```python
from build123d import *

# Parameters (mm, degrees)
BOSS_EXTRUDE1_DEPTH = 60
FILLET1_R           = 20
FILLET2_R           = 50
SKETCH2_W           = 946.025641026
SKETCH2_H           = 25
CUT_EXTRUDE1_DEPTH  = 1147.843494118
FILLET3_R           = 15
BOSS_EXTRUDE2_DEPTH = 60
CHAMFER1_START      = 58.356662002
CHAMFER1_OUTLINE_W  = 43
CHAMFER1_OUTLINE_H  = 66
CHAMFER1_DEPTH      = 20.643337998
CHAMFER2_START      = 58.356662002
CHAMFER2_OUTLINE_W  = 43
CHAMFER2_OUTLINE_H  = 66
CHAMFER2_DEPTH      = 20.643337998
FILLET4_R           = 1


with BuildPart() as part:
    # Sketch1 → Boss-Extrude1 (new, symmetric)
    with BuildSketch(Plane.XY):
        Polygon((0, 0), (0, -525), (-985, -525), (-985, -536), (-765, -575), (40, -575), (40, 0), align=None)
    extrude(amount=BOSS_EXTRUDE1_DEPTH, both=True)

    # Fillet1
    fillet1_edges = [part.edges().sort_by_distance(p)[0] for p in [
        (0, -525, 0),
    ]]
    fillet(fillet1_edges, radius=FILLET1_R)

    # Fillet2
    fillet2_edges = [part.edges().sort_by_distance(p)[0] for p in [
        (40, -575, 0),
    ]]
    fillet(fillet2_edges, radius=FILLET2_R)

    # Sketch2 → Cut-Extrude1 (cut, through all)
    with BuildSketch(Plane.XY.offset(60)):
        with Locations((-433.012820513, -562.5)):
            Rectangle(SKETCH2_W, SKETCH2_H)
    extrude(amount=-CUT_EXTRUDE1_DEPTH, mode=Mode.SUBTRACT)

    # Fillet3
    fillet3_edges = [part.edges().sort_by_distance(p)[0] for p in [
        (-985, -530.5, 60),
        (-985, -530.5, -60),
    ]]
    fillet(fillet3_edges, radius=FILLET3_R)

    # Sketch4 → Boss-Extrude2 (add, symmetric)
    with BuildSketch(Plane.XY):
        Polygon((40, -23), (71, -23), (71, -83), (62, -83), (56.90441672, -69), (40, -69), align=None)
        Polygon((40, -484), (51.812506017, -484), (58, -467), (70, -467), (70, -477), (60.172803675, -504), (40, -504), align=None)
    extrude(amount=BOSS_EXTRUDE2_DEPTH, both=True)

    # Chamfer1: read off the stored shape, not the designer's step
    # Chamfer1 outline → Chamfer1 (cut)
    with BuildSketch(Plane(origin=(0, 0, 0), x_dir=(0.7514973063417119, -0.31591606508632464, -0.5791794526582624), z_dir=(0.659736158294474, 0.35985608634244, 0.659736158294474)).offset(CHAMFER1_START)):
        with Locations((23.5, -66)):
            Rectangle(CHAMFER1_OUTLINE_W, CHAMFER1_OUTLINE_H)
    extrude(amount=CHAMFER1_DEPTH, mode=Mode.SUBTRACT)

    # Chamfer2: read off the stored shape, not the designer's step
    # Chamfer2 outline → Chamfer2 (cut)
    with BuildSketch(Plane(origin=(0, 0, 0), x_dir=(0.7514973063417119, -0.31591606508632464, 0.5791794526582624), z_dir=(0.659736158294474, 0.35985608634244, -0.659736158294474)).offset(CHAMFER2_START)):
        with Locations((23.5, 66)):
            Rectangle(CHAMFER2_OUTLINE_W, CHAMFER2_OUTLINE_H)
    extrude(amount=CHAMFER2_DEPTH, mode=Mode.SUBTRACT)

    # Fillet4
    fillet4_edges = [part.edges().sort_by_distance(p)[0] for p in [
        (56, -50.5, 60),
        (71, -23, 0),
        (71, -50.5, 45),
        (56, -23, 45),
        (56, -23, -45),
        (71, -50.5, -45),
        (56, -50.5, -60),
        (71, -83, 0),
        (40, -504, 0),
        (60.172803675, -504, 0),
        (70, -477, 0),
        (70, -467, 0),
    ]]
    fillet(fillet4_edges, radius=FILLET4_R)


solid = part.part
```
Build history of the part. All positions in model axes, mm. A direction names the side the tool comes from. Coordinates: 2 decimals unless noted, no trailing zeros. Order: outer loops, then holes, each group sorted by start corner. A loop starts at its lowest first (then second) coordinate and runs counter-clockwise, first axis right, second up.
Item 1: Tool access for faces 1 (the flat face through (-496, -525, 1)), 2 (the flat face through (40, -515, 1)), 3 (the flat face through (51, -23, -1)): list every direction of +Z, -Z, +X, -X, +Y, -Y with a clear straight run to the whole face (end or side of a thin tool).
Filled in:
face 1: +Z, -Z, -X, +Y
face 2: +Z, -Z, +X, -Y
face 3: +Z, -Z, +X, +Y
Item 2: Saw through at B-B on y = -345. List the corners of the cut face in (x, z), then the cut area to 3 significant figures.
Filled in:
outline: (0, -60) - (40, -60) - (40, 60) - (0, 60) - close
area: 4,800 mm2
Item 3: Drill centre lines: L1, parallel to X at y = -241, z = 27; L2, parallel to Y at x = -677.5, z = 0.5; L3, parallel to X at y = -57, z = -10. Where is each one in solid material? Low to high.
Filled in:
L1: x = 0 to 40
L2: y = -550 to -525
L3: x = 0 to 71
Item 4: Saw through at A-A on z = -14.5. List the corners of the cut face in (x, y), then the cut area to 3 significant figures.
Filled in:
outline: (-985, -536) - (-906.03, -550) - (33.3, -550) arc R50 ccw to (40, -525) - (40, -505) arc R1 cw to (41, -504) - (59.47, -504) arc R1 ccw to (60.41, -503.34) - (69.94, -477.17) arc R1 ccw to (70, -476.82) - (70, -468) arc R1 ccw to (69, -467) - (58, -467) - (51.81, -484) - (40, -484) - (40, -69) - (56.9, -69) - (62, -83) - (70, -83) arc R1 ccw to (71, -82) - (71, -24) arc R1 ccw to (70, -23) - (40, -23) - (40, 0) - (0, 0) - (0, -505) arc R20 cw to (-20, -525) - (-985, -525) - close
area: 48,400 mm2
Item 5: Drop flat-ended pins along their axis: pin 1 Ø8 at (x, z) = (-527, 13.5) entering from +Y; pin 2 Ø9 at (x, z) = (46.5, 21) entering from -Y; pin 3 Ø5 at (y, z) = (-75, 1) entering from -X. Give the stop position or say it passes through.
Filled in:
pin 1: stops at y = -525
pin 2: stops at y = -504
pin 3: stops at x = 0
Item 6: Saw through at C-C on x = -612. List the corners of the cut face in (y, z), then the cut area to 3 significant figures.
Filled in:
outline: (-550, -60) - (-525, -60) - (-525, 60) - (-550, 60) - close
area: 3,000 mm2
